Check sheet for the drawn part. Datum: minimum x, y, z corner. Units: mm. A direction names the side the tool comes from. Round coordinates to 2 decimals unless told otherwise and drop trailing zeros. Order: outer loops, then holes, each group sorted by start corner. A loop starts at its lowest first (then second) coordinate and runs counter-clockwise, first axis right, second up. Notation, with made-up numbers: M -22.5,64.25 L 21.5,64.25 A20 cw 21.5,86.25 Z; hole C 43.25,68 d7. An arc over 180 degrees is marked long. Use one line per item in the form item = value. Start each with the question number.
Item 1: Tool access check on the marked faces 1 and 2. Record the directions out of +Z, -Z, +X, -X, +Y, -Y that give a thin tool (end or side, any length) a straight path to the whole face; none if there is none.
Item 2: Cross-section at A-A on y = 41.5. Enter the section's corners in (x, z).
Item 3: Cross-section at C-C on y = 22.5. Count the separate pieces of the cut face and the enclosed holes in it, then the cut area to 3 significant figures.
Item 4: Thickness scan on probe 1 along Y at (x, z) = (22.5, 101.3); probe 2 along Y at (x, z) = (22, 102); probe 3 along Z at (x, y) = (7, 31.5). Record the ranges inside material, lowest first. Write a range as [from, to].
Item 5: Go/stop test with flat-tipped pins: pin 1 Ø3 at (x, z) = (22.5, 20) entering from +Y; pin 2 Ø4 at (x, z) = (37, 45.5) entering from +Y; pin 3 Ø6 at (x, z) = (34, 31) entering from +Y. Record where each tip stops, or that it passes through.
Item 6: Cross-section at D-D on z = 67. Enter the section's corners in (x, y), then the cut area to 3 significant figures.
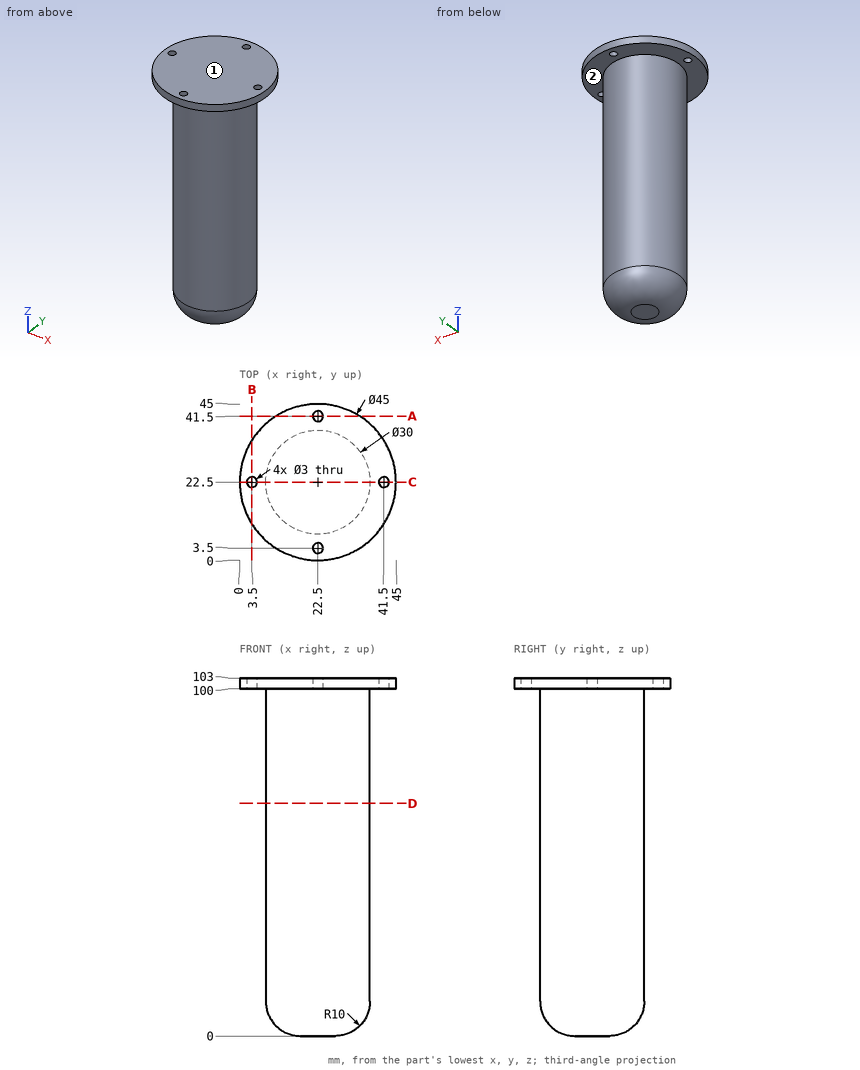
Output values:
q1.face_1 = +Z, +X, -X, +Y, -Y
q1.face_2 = -Z
q2.outline = M 10.45,100 L 21,100 L 21,103 L 10.45,103 Z; M 24,100 L 34.55,100 L 34.55,103 L 24,103 Z
q3.separate_pieces = 3
q3.enclosed_holes = 0
q3.area = 3,070 mm2
q4.probe_1 = [0, 2], [5, 40], [43, 45]
q4.probe_2 = [0.01, 2.09], [4.91, 40.09], [42.91, 44.99]
q4.probe_3 = [100, 103]
q5.pin_1 = 37.5
q5.pin_2 = 30.79
q5.pin_3 = 34.86
q6.outline = C 22.5,22.5 d30
q6.area = 707 mm2
